Geometry check sheet. Reference: the model listing, model coordinates, mm. A direction names the side the tool comes from. Coordinates: 2 decimals unless noted, no trailing zeros. Loops run counter-clockwise (first coordinate to the right, second up) from the corner with the lowest first, then second, coordinate; pieces in that order, holes last.
from build123d import *

# Parameters (mm, degrees)
F2_R     = 8.2875
F3_DEPTH = 25


# Not quite as in the source:
# - a feature names something its author has since deleted; it is built from what else it names


with BuildPart() as f1:
    # F0 (on Right) → F1 (revolve)
    with BuildSketch(Plane.YZ):
        Polygon((0, 8.2875), (0, 3), (-19.4, 3), (-20, 2.4), (-20, 0), (4, 0), (4, 8.2875), align=None)
    revolve(axis=Axis((0, -8, 0), (0, -1, 0)))

    # F2 (on face) → F3 (cut)
    with BuildSketch(Plane(origin=(0, 4, 0), x_dir=(-1, 0, 0), z_dir=(0, 1, 0))):
        Circle(F2_R)
        with BuildLine():
            ThreePointArc((0.803173326, -5.3097903559), (0, -5.525), (-0.803173326, -5.3097903559))
            Line((-0.803173326, -5.3097903559), (-4.196826674, -3.3504636819))
            ThreePointArc((-4.196826674, -3.3504636819), (-4.7847903559, -2.7625), (-5, -1.959326674))
            Line((-5, -1.959326674), (-5, 1.959326674))
            ThreePointArc((-5, 1.959326674), (-4.7847903559, 2.7625), (-4.196826674, 3.3504636819))
            Line((-4.196826674, 3.3504636819), (-0.803173326, 5.3097903559))
            ThreePointArc((-0.803173326, 5.3097903559), (0, 5.525), (0.803173326, 5.3097903559))
            Line((0.803173326, 5.3097903559), (4.196826674, 3.3504636819))
            ThreePointArc((4.196826674, 3.3504636819), (4.7847903559, 2.7625), (5, 1.959326674))
            Line((5, 1.959326674), (5, -1.959326674))
            ThreePointArc((5, -1.959326674), (4.7847903559, -2.7625), (4.196826674, -3.3504636819))
            Line((4.196826674, -3.3504636819), (0.803173326, -5.3097903559))
        make_face(mode=Mode.SUBTRACT)
    extrude(amount=-F3_DEPTH, mode=Mode.SUBTRACT)


solid = f1.part
(1) Access from +Z, -Z, +X, -X, +Y, -Y to the whole of each face (thin tool, end or side, straight path). Record for faces 1 (the cylindrical face through (0, -10, -3)), 2 (the cylindrical face through (-4.78, 2.03, 2.77)).
Findings:
face 1: -Y
face 2: +Z, -X, +Y, -Y
(2) Sectioned sample at C-C on y = -6.25. Record the cut outline in (x, z), and give its area (3 significant figures).
Findings:
outline: circle Ø6 at (0, 0)
area: 28.3 mm2
(3) Sectioned sample at A-A on z = 0. Record the cut outline in (x, y), and give its area (3 significant figures).
Findings:
outline: (-5, 0) - (-3, 0) - (-3, -19.4) - (-2.4, -20) - (2.4, -20) - (3, -19.4) - (3, 0) - (5, 0) - (5, 4) - (-5, 4) - close
area: 160 mm2
(4) Gauge pin test, flat ends, axial feed: pin 1 Ø1.5 at (x, y) = (3, 1) entering from +Z; pin 2 Ø6 at (x, y) = (3, -5) entering from -Z; pin 3 Ø2 at (y, z) = (-2, -1) entering from +X. Record the tip position at first contact, or that the pin passes through.
Findings:
pin 1: stops at z = 4.47
pin 2: stops at z = -3
pin 3: stops at x = 3
(5) Scan lines: L1, parallel to Y at x = -0.75, z = 4.25; L2, parallel to Z at x = 0, y = -17.75; L3, parallel to Z at x = -1, y = -16.75. Record each from-to range of solid material in increasing order.
Findings:
L1: y = 0 to 4
L2: z = -3 to 3
L3: z = -2.83 to 2.83
(6) Sectioned sample at B-B on x = 0. Record the cut outline in (y, z) (3 decimals).
Findings:
outline: (-20, -2.4) - (-19.4, -3) - (0, -3) - (0, -5.525) - (4, -5.525) - (4, 5.525) - (0, 5.525) - (0, 3) - (-19.4, 3) - (-20, 2.4) - close
(7) Sectioned sample at D-D on x = 3.5. Record the cut outline in (y, z).
Findings:
outline: (0, -3.75) - (4, -3.75) - (4, 3.75) - (0, 3.75) - close
